Autodesk Inventor part; units mm, degrees
ref_plane "YZ Plane" through (0, 0, 0) normal (1, 0, 0) x (0, 1, 0)
ref_plane "XZ Plane" through (0, 0, 0) normal (0, 1, 0) x (-1, 0, 0)
ref_plane "XY Plane" through (0, 0, 0) normal (0, 0, 1) x (1, 0, 0)
sketch "Sketch1" plane through (0, 0, 0) normal (0, 0, 1) x (1, 0, 0)
  line L0 (-750, 67.4521) -> (750, 67.4521)
  line L1 (750, 67.4521) -> (750, 0)
  line L2 (750, 0) -> (-750, 0)
  line L3 (-750, 0) -> (-750, 67.4521)
  point P0 (0, 0)
  point P1 (0, 0)
  dimension "d0" = 1500
  dimension "d1" = 67.4521
extrude "Plate1" add sketch "Sketch1" along normal blind 2
sketch "Sketch2" plane through (750, 2, 0) normal (0, -1, 0) x (1, 0, 0)
  line L0 (-1500, 0) -> (0, 0)
  line L1 (0, 0) -> (0, 30)
  line L2 (0, 30) -> (-1500, 30)
  line L3 (-1500, 30) -> (-1500, 0)
edge flange "Flange1" height 30 angle 90 thickness 2 bend radius 2 thickness toward (0, -1, 0) relief tear relief width 2 relief depth 1 edges at (0, 0, 2) wall of the first edge with corners at (-750, 2, 0) (750, 2, 0) (750, 2, 30) (-750, 2, 30)
bend "Bend1"
corner "Corner1"
sketch "Sketch5" plane through (0, 0, 0) normal (0, 0, -1) x (-1, 0, 0)
  line L0 (750, 67.4521) -> (-750, 67.4521)
  line L1 (499, 67.4521) -> (499, 29)
  line L2 (499, 29) -> (501, 29)
  line L3 (501, 29) -> (501, 67.4521)
  line L4 (750, 0) -> (-750, 0)
  point P0 (0, 0)
  point P1 (500, 29)
  dimension "d18" = 2
  dimension "d20" = 29
  dimension "d27" = 250
extrude "Extrusion1" cut sketch "Sketch5" against normal through all
pattern_linear "Rectangular Pattern1" count 3 spacing 500 along (1, 0, 0) of "Extrusion1"
sketch "Sketch6" plane through (0, 0, 0) normal (0, 0, -1) x (-1, 0, 0)
  line L0 (-750, 67.4521) -> (-750, 4)
  circle A0 centre (-750, 67.4521) radius 15
  line L1 (-750, 67.4521) -> (-501, 67.4521)
  point P0 (0, 0)
  point P1 (-735, 67.4521)
  point P2 (-750, 52.4521)
  dimension "d24" = 30
extrude "Extrusion2" cut sketch "Sketch6" against normal through all contours L1 A0 L0 picked at (-740.1254, 66.3395)
mirror "Mirror1" about plane through (0, 0, 0) normal (1, 0, 0) of "Extrusion2"
equation "\"d1\" = Стрингер_2"
equation "\"d18\" = Thickness"
equation "\"d2\" = Thickness"
equation "\"d3\" = BendReliefWidth"
equation "\"d4\" = BendReliefDepth"
equation "\"d5\" = MinimumRemnant"
equation "\"d6\" = TransitionRadius"
equation "\"d9\" = BendRadius"
equation "\"d10\" = CornerReliefSize"
equation "\"d11\" = GapSize"
equation "\"d12\" = JacobiRadiusSize"
equation "\"BendRadius\" = Thickness"
equation "\"BendReliefWidth\" = Thickness"
equation "\"BendReliefDepth\" = 0.5 * Thickness"
equation "\"CornerReliefSize\" = 4 * Thickness"
equation "\"MinimumRemnant\" = 2 * Thickness"
equation "\"TransitionRadius\" = BendRadius"
equation "\"JacobiRadiusSize\" = BendRadius"
equation "\"GapSize\" = Thickness"
equation "\"qqqqqq\" = 67.35706"
properties part number "МОО 052 стрингер спина 21" material "Stainless Steel"
Geometry check sheet. Reference: the model listing, model coordinates, mm. A direction names the side the tool comes from. Round coordinates to 2 decimals unless told otherwise and drop trailing zeros. Loops run counter-clockwise (first coordinate to the right, second up) from the corner with the lowest first, then second, coordinate; pieces in that order, holes last. Notation, with made-up numbers: (-27, -24.5) - (30, -24.5) arc R9 ccw to (30, -8.5) - close; hole circle Ø1 at (23.25, 0.25). An arc over 180 degrees is marked (long way). Write each question's results on one line, items separated by ' | '. Start each with the question number.
Q1. Thickness scan on line 1 (X direction, y = 41, z = 1.5); line 2 (Y direction, x = -526, z = 27.75). Record the ranges inside material, lowest first. Write a range as [from, to].
Q2. Access from +Z, -Z, +X, -X, +Y, -Y to the whole of each face (thin tool, end or side, straight path). Record for faces 1 (the flat face through (-10, 36, 2)), 2 (the flat face through (750, 18.3, 1.7)).
Q3. Cross-section at B-B on z = 10.25. Enter the section's corners in (x, y), and give its area (3 significant figures).
Q4. Gauge pin test, flat ends, axial feed: P1, Ø1, axis at x = -503, z = 22, coming from the +Y side; P2, Ø6, axis at y = 16.5, z = 6, coming from the -X side; P3, Ø2, axis at x = -342, y = 10, coming from the +Z side; P4, Ø1, axis at x = -500, z = 0.5, coming from the +Y side. Record the tip position at first contact, or that the pin passes through.
Q5. Cross-section at A-A on x = 443. Enter the section's corners in (y, z), and give its area (3 significant figures).
Answers below:
1) line 1: x = [-750, -501], [-499, -1], [1, 499], [501, 750] | line 2: y = [0, 2]
2) face 1: +Z, +X, -X, +Y | face 2: +Z, -Z, +X, +Y, -Y
3) outline: (-750, 0) - (750, 0) - (750, 2) - (-750, 2) - close | area: 3,000 mm²
4) P1: stops at y = 2 | P2: passes through | P3: stops at z = 2 | P4: stops at y = 29
5) outline: (0, 4) arc R4 ccw to (4, 0) - (67.45, 0) - (67.45, 2) - (4, 2) arc R2 cw to (2, 4) - (2, 30) - (0, 30) - close | area: 188 mm²
